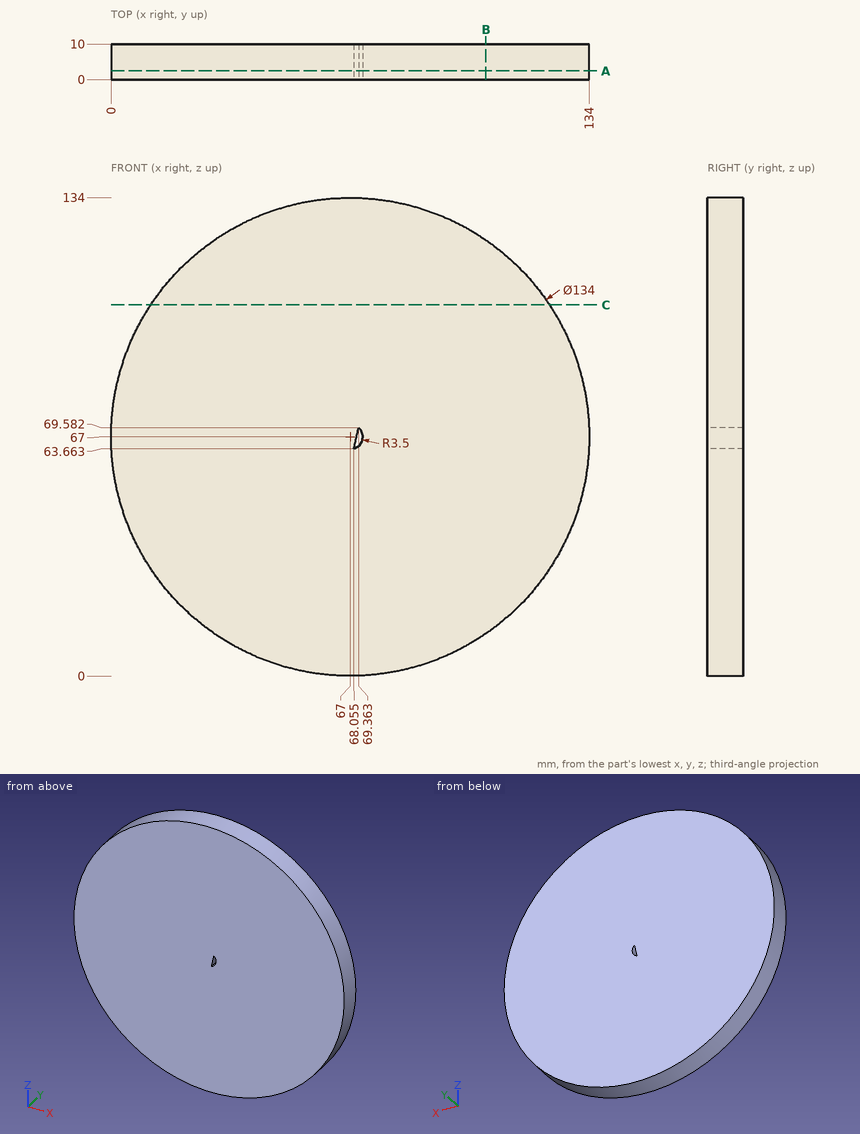
Source: three-view drawing plus pictorial views. Frame: mm from the lowest corner of the part. Coordinates: 2 decimals unless noted, no trailing zeros. Loops run counter-clockwise (first coordinate to the right, second up) from the corner with the lowest first, then second, coordinate; pieces in that order, holes last. Notation, with made-up numbers: (30, 84) - (72, 84) arc R10 cw to (72, 94) - close; hole circle Ø5 at (-37, 51). An arc over 180 degrees is marked (long way). One line per question, with ' | ' between items.
1) Section C-C, the plane z = 104. Return loops of the section in (x, y).
Report:
outline: (11.14, 0) - (122.86, 0) - (122.86, 10) - (11.14, 10) - close
2) Line query: line 1 along X through (y, z) = (1.5, 66.5); line 2 along X through (y, z) = (5, 69) (1 decimal); line 3 along X through (y, z) = (9.25, 20.5) (1 decimal). Output: solid intervals per line, ascending.
Report:
line 1: x = 0 to 68.68, 70.46 to 134 | line 2: x = 0 to 69.2, 69.9 to 134 | line 3: x = 18.8 to 115.2
3) Section A-A, the plane y = 2.5. Return loops of the section in (x, z) (1 decimal), then the cut area to 3 significant figures.
Report:
outline: circle Ø134 at (67, 67); hole (68.1, 63.7) arc R3.5 ccw to (69.4, 69.6) - close | area: 14,100 mm²
4) First-contact query: P1, Ø1.5, axis at x = 92, y = 8.5, coming from the +Z side; P2, Ø3, axis at y = 4.5, z = 57.5, coming from the -X side; P3, Ø2, axis at y = 3, z = 112, coming from the +X side. Flat tips, straight axial feed; report the tip coordinate or a pass-through.
Report:
P1: stops at z = 129.46 | P2: stops at x = 0.48 | P3: stops at x = 117.53
5) Section B-B, the plane x = 105. Return loops of the section in (y, z), then the cut area to 3 significant figures.
Report:
outline: (0, 11.82) - (10, 11.82) - (10, 122.18) - (0, 122.18) - close | area: 1,100 mm²
